Geometry check sheet. Reference: the model listing, model coordinates, mm. Face numbers are marked on the shaded views. Give positions to 0.01 mm unless a question says otherwise; leave off trailing zeros. Loops run counter-clockwise (first coordinate to the right, second up) from the corner with the lowest first, then second, coordinate; pieces in that order, holes last. Notation, with made-up numbers: (2, 12) -> (58, 12) arc R26 cw to (58, 32) -> close; hole circle Ø1 at (37, 0.25). An arc over 180 degrees is marked (long way). Answer as a JSON object with one key per item and string values.
Autodesk Inventor part; units mm, degrees
ref_plane "YZ Plane" through (0, 0, 0) normal (1, 0, 0) x (0, 1, 0)
ref_plane "XZ Plane" through (0, 0, 0) normal (0, 1, 0) x (-1, 0, 0)
ref_plane "XY Plane" through (0, 0, 0) normal (0, 0, 1) x (1, 0, 0)
sketch "Sketch1" plane through (0, 0, 0) normal (1, 0, 0) x (0, 1, 0)
  line L0 (-100, -33.2) -> (50, -33.2)
  line L1 (50, -33.2) -> (50, -34.3)
  line L2 (-100, -34.2) -> (-100, -33.2)
  line L3 (100, -34.3) -> (100, -35.3)
  line L4 (100, -35.3) -> (-50, -35.3)
  line L5 (-140, 0) -> (140, 0)
  line L6 (100, -34.3) -> (50, -34.3)
  line L7 (-100, -34.2) -> (-50, -34.2)
  line L8 (-50, -34.2) -> (-50, -35.3)
  point P0 (0, 0)
  point P1 (-100, -33.875)
  point P2 (100, -34.75)
  dimension "d6" = 33.2
  dimension "d7" = 50
  dimension "d9" = 200
  dimension "d13" = 2.1
  dimension "d16" = 100
  dimension "d26" = 1
  dimension "d27" = 1
  dimension "d28" = 34.3
  dimension "d29" = 34.2
revolve "Revolution1" add sketch "Sketch1" angle 360 about axis through (0, -10, 0) along (0, 1, 0)
sketch "Sketch2" plane through (0, 0, 0) normal (1, 0, 0) x (0, 1, 0)
  line L0 (71, 3) -> (65, 3)
  line L1 (65, 3) -> (65, -3)
  line L2 (65, -3) -> (71, -3)
  line L3 (71, -3) -> (71, 3)
  line L4 (100, -35.3) -> (100, 35.3)
  point P0 (0, 0)
  dimension "d17" = 3
  dimension "d18" = 3
  dimension "d19" = 6
  dimension "d20" = 29
extrude "Extrusion1" [suppressed]
equation "\"gap\" = 0.1"
properties part number "MidTube"
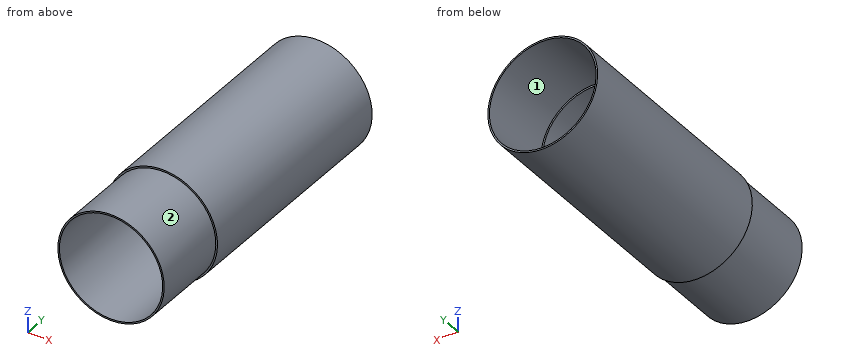
1) Section check C-C on y = -75.5. Record the cut outline in (x, z).
Geometry check:
{"outline": "circle Ø68.4 at (0, 0); hole circle Ø66.4 at (0, 0)"}
2) Section check A-A on z = 0. Record the cut outline in (x, y), plus the area to 3 significant figures.
Geometry check:
{"outline": "(-35.3, -50) -> (-34.2, -50) -> (-34.2, -100) -> (-33.2, -100) -> (-33.2, 50) -> (-34.3, 50) -> (-34.3, 100) -> (-35.3, 100) -> close; (33.2, -100) -> (34.2, -100) -> (34.2, -50) -> (35.3, -50) -> (35.3, 100) -> (34.3, 100) -> (34.3, 50) -> (33.2, 50) -> close", "area": "620 mm2"}
3) Draft check along X on the marked faces 1 and 2. Enter one of: pulls with the +X half, pulls with the -X half, needs draft (parallel to the pull), parting line crosses it, or undercut.
Geometry check:
{"face 1": "undercut", "face 2": "parting line crosses it"}
4) Depth check by flat-ended pin: P1, Ø8, axis at y = 9, z = 4.5, coming from the +X side; P2, Ø4, axis at y = 35, z = -10, coming from the -X side; P3, Ø1.5, axis at x = -17, y = 25.5, coming from the -Z side. Enter the tip coordinate at first touch or a pass-through.
Geometry check:
{"P1": "stops at x = 35.3", "P2": "stops at x = -34.38", "P3": "stops at z = -31.34"}
5) Section check D-D on y = 31.5. Record the cut outline in (x, z).
Geometry check:
{"outline": "circle Ø70.6 at (0, 0); hole circle Ø66.4 at (0, 0)"}
6) Section check B-B on x = 0. Record the cut outline in (y, z).
Geometry check:
{"outline": "(-100, -34.2) -> (-50, -34.2) -> (-50, -35.3) -> (100, -35.3) -> (100, -34.3) -> (50, -34.3) -> (50, -33.2) -> (-100, -33.2) -> close; (-100, 33.2) -> (50, 33.2) -> (50, 34.3) -> (100, 34.3) -> (100, 35.3) -> (-50, 35.3) -> (-50, 34.2) -> (-100, 34.2) -> close"}
7) Material ranges on line 1 along Z through (x, y) = (0, 77); line 2 along X through (y, z) = (-66, 0); line 3 along X through (y, z) = (-21, 1.5), recorded low to high. Write a range as from..to.
Geometry check:
{"line 1": "z = -35.3..-34.3, 34.3..35.3", "line 2": "x = -34.2..-33.2, 33.2..34.2", "line 3": "x = -35.27..-33.17, 33.17..35.27"}
